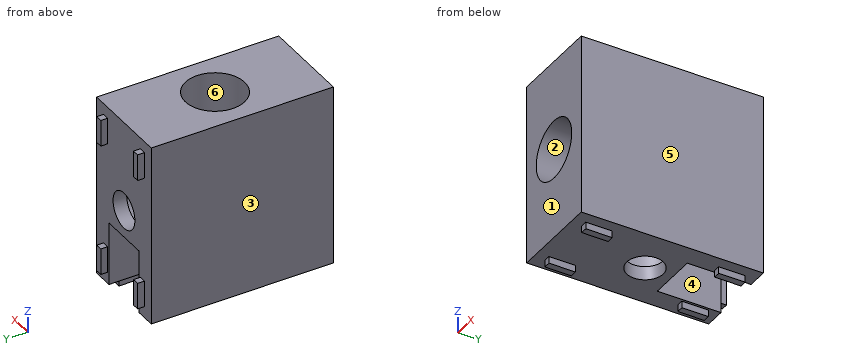
from build123d import *

# Parameters (mm, degrees)
SKETCH_2_W               = 40
SKETCH_2_H               = 40
EXTRUDE_2_DEPTH          = 10
SKETCH_4_W               = 1.5
SKETCH_4_H               = 5.8
EXTRUDE_3_DEPTH          = 1.5
SKETCH_5_W               = 14
SKETCH_5_H               = 14
CUT_EXTRUDE_1_DEPTH      = 5.5
CUT_EXTRUDE_1_DEPTH_BACK = 5.5


with BuildPart() as part:
    # Эскиз2 → Бобышка-Вытянуть2 (new body, symmetric)
    with BuildSketch(Plane(origin=(0, 0, 0), x_dir=(0, 0, -1), z_dir=(1, 0, 0))):
        Rectangle(SKETCH_2_W, SKETCH_2_H)
    extrude(amount=EXTRUDE_2_DEPTH, both=True)

    # Эскиз3 → Вырез-Повернуть1 (revolve, cut)
    with BuildSketch(Plane.XY, mode=Mode.PRIVATE) as cut_revolve_1_sk:
        Polygon((-4, 20), (-4, 17), (-6.5, 17), (-6.5, -20), (0, -20), (0, 20), align=None)
    cut_revolve_1 = revolve(cut_revolve_1_sk.sketch.rotate(Axis((0, -20, 0), (0, 1, 0)), 180), axis=Axis((0, -20, 0), (0, 1, 0)), mode=Mode.SUBTRACT)  # turned: the seam where the file's is

    # Эскиз4 → Бобышка-Вытянуть3 (add)
    with BuildSketch(Plane(origin=(0, 20, 0), x_dir=(1, 0, 0), z_dir=(0, 1, 0))):
        with Locations((-6.75, -14.6)):
            Rectangle(SKETCH_4_W, SKETCH_4_H)
        with Locations((-6.75, 14.6)):
            Rectangle(SKETCH_4_W, SKETCH_4_H)
        with Locations((6.75, 14.6)):
            Rectangle(SKETCH_4_W, SKETCH_4_H)
        with Locations((6.75, -14.6)):
            Rectangle(SKETCH_4_W, SKETCH_4_H)
    extrude_3 = extrude(amount=EXTRUDE_3_DEPTH)

    # Зеркальное отражение1: Вырез-Повернуть1, Бобышка-Вытянуть3 across plane
    add(cut_revolve_1.mirror(Plane(origin=(0, 0, 0), x_dir=(0, -0.707106781, 0.707106781), z_dir=(0, 0.707106781, 0.707106781))), mode=Mode.SUBTRACT)
    add(extrude_3.mirror(Plane(origin=(0, 0, 0), x_dir=(0, -0.707106781, 0.707106781), z_dir=(0, 0.707106781, 0.707106781))))

    # Эскиз5 → Вырез-Вытянуть1 (cut, two sides)
    with BuildSketch(Plane(origin=(0, 0, 0), x_dir=(0, 0, -1), z_dir=(1, 0, 0))) as cut_extrude_1_sk:
        with Locations((13, 13)):
            Rectangle(SKETCH_5_W, SKETCH_5_H)
    extrude(amount=CUT_EXTRUDE_1_DEPTH, mode=Mode.SUBTRACT)
    extrude(cut_extrude_1_sk.sketch, amount=-CUT_EXTRUDE_1_DEPTH_BACK, mode=Mode.SUBTRACT)


solid = part.part
Build history of the part. All positions in model axes, mm. Face numbers are marked on the shaded views. A direction names the side the tool comes from. Round coordinates to 2 decimals unless told otherwise and drop trailing zeros. Write each loop counter-clockwise with the first axis right and the second up, starting at its lowest first coordinate (ties: lowest second). Pieces come first, ordered by that corner, then holes. Notation, with made-up numbers: (-17.5, 70) -> (18.5, 70) arc R10 ccw to (18.5, 78) -> close; hole circle Ø7 at (9.5, 39.5). An arc over 180 degrees is marked (long way). Use one line per item in the form item = value.
Q1. Band-saw the part on D-D, the plane z = -8. Write the cut outline in (x, y), then the cut area to 3 significant figures.
Conclusion:
outline = (-10, -20) -> (10, -20) -> (10, 20) -> (5.5, 20) -> (5.5, 6) -> (2.5, 6) arc R6.5 cw (long way) to (-2.5, 6) -> (-5.5, 6) -> (-5.5, 20) -> (-10, 20) -> close
area = 515 mm²
Q2. Two-plate mould, pull along X, no slides. Class the marked faces 1, 2 and 3: released by +X, released by -X, zero draft, split by the parting line, or undercut.
Conclusion:
face_1 = zero draft
face_2 = undercut
face_3 = released by -X
Q3. Band-saw the part on A-A, the plane x = 0. Write the cut outline in (y, z).
Conclusion:
outline = (-20, -20) -> (-4, -20) -> (-4, -17) -> (-6.5, -17) -> (-6.5, -6.5) -> (-20, -6.5) -> close; (-20, 6.5) -> (-6.5, 6.5) -> (-6.5, 20) -> (-20, 20) -> close; (4, -20) -> (6, -20) -> (6, -17) -> (4, -17) -> close; (6.5, 6.5) -> (17, 6.5) -> (17, 4) -> (20, 4) -> (20, 20) -> (6.5, 20) -> close; (17, -6) -> (20, -6) -> (20, -4) -> (17, -4) -> close
Q4. Tool access for the marked faces 4, 5 and 6: list every direction of +Z, -Z, +X, -X, +Y, -Y with a clear straight run to the whole face (end or side of a thin tool).
Conclusion:
face_4 = -Z, +Y
face_5 = +Z, -Z, +X, +Y, -Y
face_6 = +Z
Q5. Drill centre lines: L1, parallel to Y at x = 0, z = 9.25; L2, parallel to Y at x = 0, z = -18.8; L3, parallel to X at y = 0, z = 11.75. Where is each one in solid material? Low to high.
Conclusion:
L1 = -20 to -6.5, 6.5 to 20
L2 = -20 to -4, 4 to 6
L3 = -10 to -6.5, 6.5 to 10
Q6. Band-saw the part on C-C, the plane y = 9.5. Write the cut outline in (x, z).
Conclusion:
outline = (-10, -20) -> (-5.5, -20) -> (-5.5, -6) -> (-2.5, -6) arc R6.5 cw (long way) to (2.5, -6) -> (5.5, -6) -> (5.5, -20) -> (10, -20) -> (10, 20) -> (-10, 20) -> close
Q7. Drop flat-ended pins along their axis: P1, Ø6.5, axis at x = 0, y = 0, coming from the -Z side; P2, Ø1.2, axis at y = 21, z = 15, coming from the -X side; P3, Ø11.5, axis at x = 0, z = 0, coming from the +Y side; P4, Ø1.6, axis at x = 6.5, y = 21, coming from the +Z side. Give the stop position or say it passes through.
Conclusion:
P1 = through
P2 = -7.5
P3 = 20
P4 = 17.5
Q8. Band-saw the part on B-B, the plane z = -3. Write the cut outline in (x, y), then the cut area to 3 significant figures.
Conclusion:
outline = (-10, -20) -> (-5.77, -20) -> (-5.77, -3) arc R6.5 cw to (-5.77, 3) -> (-5.77, 17) -> (-2.65, 17) -> (-2.65, 20) -> (-10, 20) -> close; (2.65, 17) -> (5.77, 17) -> (5.77, 3) arc R6.5 cw to (5.77, -3) -> (5.77, -20) -> (10, -20) -> (10, 20) -> (2.65, 20) -> close
area = 351 mm²
